Check sheet for the drawn part. Datum: minimum x, y, z corner. Units: mm. A direction names the side the tool comes from. Give positions to 0.01 mm unless a question says otherwise; leave off trailing zeros. Loops run counter-clockwise (first coordinate to the right, second up) from the corner with the lowest first, then second, coordinate; pieces in that order, holes last. Notation, with made-up numbers: M 70,17.25 L 92,17.25 A16 cw 92,41.25 Z; hole C 33.25,-25 d8. An arc over 180 degrees is marked long. Write each question's results on one line, items separated by ' | '. Start each with the question number.
1. Sectioned sample at D-D on z = 22. Record the cut outline in (x, y), and give its area (3 significant figures).
2. Tool access check on the marked faces 5, 6 and 7. Record the directions out of +Z, -Z, +X, -X, +Y, -Y that give a thin tool (end or side, any length) a straight path to the whole face; none if there is none.
3. Go/stop test with flat-tipped pins: pin 1 (5 mm diameter, centred on x = 9, y = 3, fed in from -Z); pin 2 (1.5 mm diameter, centred on y = 7.5, z = 43, fed in from -X); pin 3 (1.5 mm diameter, centred on y = 6.5, z = 41, fed in from +X). Record where each tip stops, or that it passes through.
4. Material ranges on line 1 along Z through (x, y) = (19.9, 3.5); line 2 along Z through (x, y) = (20, 4); line 3 along Y through (x, z) = (19.9, 41.75), recorded low to high.
5. Draft check along Z on the marked faces 1, 2, 3 and 4. Enter one of: pulls with the +Z half, pulls with the -Z half, needs draft (parallel to the pull), parting line crosses it, or undercut.
6. Sectioned sample at B-B on y = 5.75. Record the cut outline in (x, z) (1 decimal).
7. Sectioned sample at A-A on x = 19.9. Record the cut outline in (y, z).
8. Sectioned sample at C-C on x = 7. Record the cut outline in (y, z).
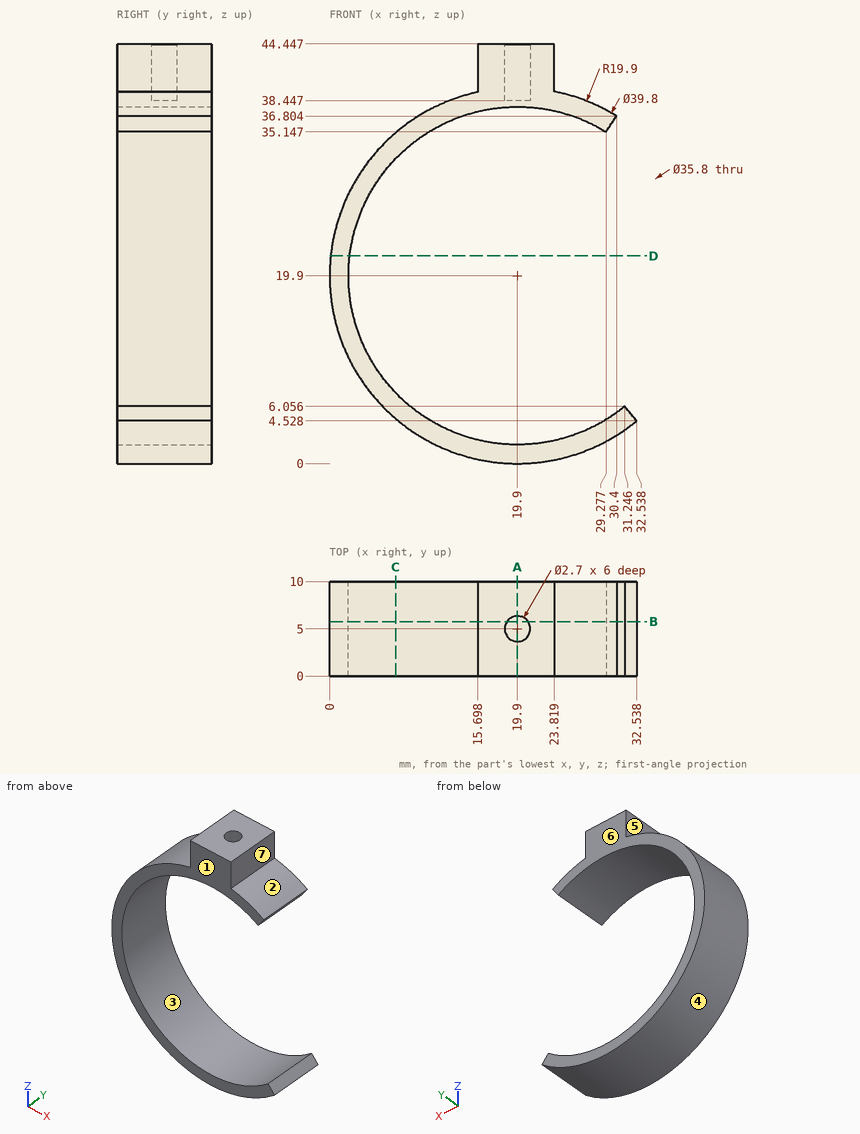
Output values:
1) outline: M 0.11,0 L 2.12,0 L 2.12,10 L 0.11,10 Z | area: 20.1 mm2
2) face 5: +Z, -X, +Y, -Y | face 6: +Z, -Z, +X, -X, +Y | face 7: +Z, +X, +Y, -Y
3) pin 1: z = 1.86 | pin 2: x = 15.7 | pin 3: x = 23.82
4) line 1: 0 to 2, 37.8 to 44.45 | line 2: 0 to 2, 37.8 to 38.45 | line 3: 0 to 3.65, 6.35 to 10
5) face 1: needs draft | face 2: pulls with the +Z half | face 3: undercut | face 4: parting line crosses it
6) outline: M 15.7,39.4 A19.9 ccw long 32.5,4.5 L 31.2,6.1 A17.9 cw long 29.3,35.1 L 30.4,36.8 A19.9 ccw 23.8,39.4 L 23.8,44.4 L 21,44.4 L 21,38.4 L 18.8,38.4 L 18.8,44.4 L 15.7,44.4 Z
7) outline: M 0,0 L 10,0 L 10,2 L 0,2 Z; M 0,37.8 L 10,37.8 L 10,44.45 L 6.35,44.45 L 6.35,38.45 L 3.65,38.45 L 3.65,44.45 L 0,44.45 Z
8) outline: M 0,4.75 L 10,4.75 L 10,7.49 L 0,7.49 Z; M 0,32.31 L 10,32.31 L 10,35.05 L 0,35.05 Z
